Read the model definition and answer for the solid it produces. Units are mm, in the model's axes. Face numbers are marked on the shaded views. Give positions to 0.01 mm unless a question says otherwise; leave off trailing zeros. Loops run counter-clockwise (first coordinate to the right, second up) from the corner with the lowest first, then second, coordinate; pieces in that order, holes last.
(1) Each of these flat-tipped pins is pushed along its axis until it touches: P1, Ø2, axis at x = 16.5, y = 17.5, coming from the +Z side; P2, Ø4.5, axis at x = 16, y = 7, coming from the +Z side. Where does it stop, or does it pass through?
(2) Straight lines are drawn through the part: probe 1 along Y at (x, z) = (30, 11.25); probe 2 along Y at (x, z) = (29.5, 9.25). For each, find the intervals that lie inside material, in ascending order.
(3) Find section C-C, the plane x = 50. Write down the section's boundary in (y, z).
(4) Find section A-A, the plane z = 8.25. State how many separate pieces and enclosed holes the cut face has, then the cut area to 3 significant figures.
(5) Determine the mould class of the marked faces 1, 2, 3 and 4 for opening direction X: pulls with the +X half, pulls with the -X half, needs draft (parallel to the pull), parting line crosses it, or undercut.
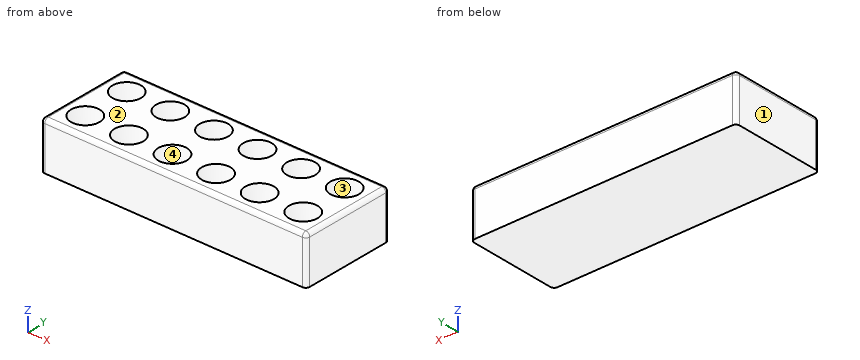
```python
from build123d import *

# Parameters (mm, degrees)
ARRAY_X_COUNT = 6
ARRAY_X_PITCH = 11
ARRAY_Y_COUNT = 2
ARRAY_Y_PITCH = 12
BOX_W         = 67
BOX_H         = 24
BOX_DEPTH     = 12
FILLET_R      = 1


with BuildPart() as array:
    # Cone → Cone (revolve)
    with BuildSketch(Plane(origin=(6, 6, 4), x_dir=(1, 0, 0), z_dir=(0, -1, 0))):
        Polygon((0, 0), (2, 0), (4, 10), (0, 10), align=None)
    revolve(axis=Axis((6, 6, 4), (0, 0, 1)))

    # Array X: Array ×6


with BuildPart() as array_1:
    add(array.part)
    with Locations(*[(i * ARRAY_X_PITCH, 0, 0) for i in range(1, ARRAY_X_COUNT)]):
        add(array.part)

    # Array Y: Array ×2


with BuildPart() as array_2:
    add(array_1.part)
    with Locations(*[(0, i * ARRAY_Y_PITCH, 0) for i in range(1, ARRAY_Y_COUNT)]):
        add(array_1.part)


with BuildPart() as cut:
    # Box → Box (new body)
    with BuildSketch(Plane.XY):
        with Locations((33.5, 12)):
            Rectangle(BOX_W, BOX_H)
    extrude(amount=BOX_DEPTH)

    # Fillet
    fillet_edges = [cut.edges().sort_by_distance(p)[0] for p in [
        (0, 0, 6),
        (0, 12, 12),
        (0, 24, 6),
        (67, 0, 6),
        (67, 12, 12),
        (67, 24, 6),
        (33.5, 0, 12),
        (33.5, 24, 12),
    ]]
    fillet(fillet_edges, radius=FILLET_R)

    # Cut: cut Array
    add(array_2.part, mode=Mode.SUBTRACT)


solid = cut.part
```
Entries:
1. P1: stops at z = 4
1. P2: stops at z = 12
2. probe 1: y = 0.03 to 3.19, 8.81 to 15.19, 20.81 to 23.97
2. probe 2: y = 0 to 3.34, 8.66 to 15.34, 20.66 to 24
3. outline: (0, 0) - (24, 0) - (24, 11) arc R1 ccw to (23, 12) - (21.6, 12) - (20, 4) - (16, 4) - (14.4, 12) - (9.6, 12) - (8, 4) - (4, 4) - (2.4, 12) - (1, 12) arc R1 ccw to (0, 11) - close
4. separate pieces: 1
4. enclosed holes: 12
4. area: 1,300 mm2
5. face 1: pulls with the -X half
5. face 2: needs draft
5. face 3: undercut
5. face 4: undercut
